```python
from build123d import *

# Parameters (mm, degrees)
SKETCH023_W         = 40
SKETCH023_H         = 45
SKETCH023_R         = 1.75
SKETCH023_R_2       = 5.15
SKETCH023_R_3       = 1.6
PAD007_DEPTH        = 4
FILLET005_R         = 3
HOLE001_D           = 3.4
HOLE001_DEPTH       = 25
HOLE001_CSINK_D     = 6.2
HOLE001_CSINK_ANGLE = 90


with BuildPart() as part:
    # Sketch023 → Pad007 (new body)
    with BuildSketch(Plane.XY):
        Rectangle(SKETCH023_W, SKETCH023_H)
        with Locations((-16, 18.5)):
            Circle(SKETCH023_R, mode=Mode.SUBTRACT)
        with Locations((16, 18.5)):
            Circle(SKETCH023_R, mode=Mode.SUBTRACT)
        with Locations((16, -18.5)):
            Circle(SKETCH023_R, mode=Mode.SUBTRACT)
        with Locations((-16, -18.5)):
            Circle(SKETCH023_R, mode=Mode.SUBTRACT)
        with Locations((0, -9.5)):
            Circle(SKETCH023_R_2, mode=Mode.SUBTRACT)
        with Locations((0, -19)):
            Circle(SKETCH023_R_3, mode=Mode.SUBTRACT)
        with Locations((-10, 10.5)):
            Circle(SKETCH023_R_3, mode=Mode.SUBTRACT)
        with Locations((10, 10.5)):
            Circle(SKETCH023_R_3, mode=Mode.SUBTRACT)
    extrude(amount=PAD007_DEPTH)

    # Fillet005
    fillet005_edges = [part.edges().sort_by_distance(p)[0] for p in [
        (20, 22.5, 2),
        (-20, -22.5, 2),
        (-20, 22.5, 2),
        (20, -22.5, 2),
    ]]
    fillet(fillet005_edges, radius=FILLET005_R)

    # Hole001
    with Locations(Plane(origin=(0, 0, 0), x_dir=(1, 0, 0), z_dir=(0, 0, -1))):
        with Locations((0, 19), (10, -10.5), (-10, -10.5)):
            CounterSinkHole(HOLE001_D / 2, HOLE001_CSINK_D / 2, depth=HOLE001_DEPTH, counter_sink_angle=HOLE001_CSINK_ANGLE)


solid = part.part
```
The model under review builds one solid part; all positions refer to its coordinate system, in mm. Round coordinates to 2 decimals unless told otherwise and drop trailing zeros. Order: outer loops, then holes, each group sorted by start corner. A loop starts at its lowest first (then second) coordinate and runs counter-clockwise, first axis right, second up. Notation, with made-up numbers: (33, 83.5) - (71, 83.5) arc R23 cw to (71, 117.5) - close; hole circle Ø7 at (45, 79). An arc over 180 degrees is marked (long way). Answer in a Markdown table with one row per item.
(1) Take a section at A-A on x = 16. Write out the cut boundary in (y, z).
Result set:
| item | result |
|---|---|
| outline | (-22.5, 0) - (-20.25, 0) - (-20.25, 4) - (-22.5, 4) - close; (-16.75, 0) - (16.75, 0) - (16.75, 4) - (-16.75, 4) - close; (20.25, 0) - (22.5, 0) - (22.5, 4) - (20.25, 4) - close |
(2) Take a section at C-C on z = 0.5. Count the separate pieces of the cut face and the enclosed holes in it, plus the area to 3 significant figures.
Result set:
| item | result |
|---|---|
| separate pieces | 1 |
| enclosed holes | 8 |
| area | 1,610 mm2 |
(3) Clearance check with flat-ended pins moving along their axes: P1, Ø12, axis at x = 12, y = 16.5, coming from the -Z side; P2, Ø2.5, axis at x = 0, y = -19, coming from the +Z side. State where each tip first meets the part, or that it passes through.
Result set:
| item | result |
|---|---|
| P1 | stops at z = 0 |
| P2 | passes through |
(4) Take a section at D-D on x = 10. Write out the cut boundary in (y, z), plus the area to 3 significant figures.
Result set:
| item | result |
|---|---|
| outline | (-22.5, 0) - (7.4, 0) - (8.8, 1.4) - (8.8, 4) - (-22.5, 4) - close; (12.2, 1.4) - (13.6, 0) - (22.5, 0) - (22.5, 4) - (12.2, 4) - close |
| area | 164 mm2 |
(5) Take a section at B-B on y = 18.5. Write out the cut boundary in (x, z).
Result set:
| item | result |
|---|---|
| outline | (-20, 0) - (-17.75, 0) - (-17.75, 4) - (-20, 4) - close; (-14.25, 0) - (14.25, 0) - (14.25, 4) - (-14.25, 4) - close; (17.75, 0) - (20, 0) - (20, 4) - (17.75, 4) - close |
(6) For line 1 (Y direction, x = 0, z = 2.15); line 2 (Y direction, x = -16, z = 1.25); line 3 (X direction, y = 12, z = 0.4) (3 decimals), list the stretches that pass through material, from the lowest coordinate up. Write a range as from..to.
Result set:
| item | result |
|---|---|
| line 1 | y = -22.5..-20.7, -17.3..-14.65, -4.35..22.5 |
| line 2 | y = -22.5..-20.25, -16.75..16.75, 20.25..22.5 |
| line 3 | x = -20..-12.245, -7.755..7.755, 12.245..20 |
